```python
from build123d import *

# Parameters (mm, degrees)
SKETCH1_W           = 199.69
SKETCH1_H           = 98.8
SKETCH1_R           = 2
BOSS_EXTRUDE1_DEPTH = 3


with BuildPart() as part:
    # Sketch1 → Boss-Extrude1 (new body)
    with BuildSketch(Plane(origin=(0, 0, 0), x_dir=(1, 0, 0), z_dir=(0, 1, 0))):
        with Locations((49.702752105, -22.572203273)):
            Rectangle(SKETCH1_W, SKETCH1_H)
        with Locations((124.547752105, -0.072203273)):
            Circle(SKETCH1_R, mode=Mode.SUBTRACT)
        with Locations((124.547752105, -45.072203273)):
            Circle(SKETCH1_R, mode=Mode.SUBTRACT)
        with BuildLine():
            Line((-41.155575491, 15.827796727), (3.397752105, 15.827796727))
            ThreePointArc((3.397752105, 15.827796727), (4.281635581, 16.193913251), (4.647752105, 17.077796727))
            Line((4.647752105, 17.077796727), (4.647752105, 17.577796727))
            ThreePointArc((4.647752105, 17.577796727), (5.013868628, 18.461680204), (5.897752105, 18.827796727))
            Line((5.897752105, 18.827796727), (15.397752105, 18.827796727))
            ThreePointArc((15.397752105, 18.827796727), (16.281635581, 18.461680204), (16.647752105, 17.577796727))
            Line((16.647752105, 17.577796727), (16.647752105, 17.077796727))
            ThreePointArc((16.647752105, 17.077796727), (17.013868628, 16.193913251), (17.897752105, 15.827796727))
            Line((17.897752105, 15.827796727), (106.2510797, 15.827796727))
            ThreePointArc((106.2510797, 15.827796727), (107.693618601, 15.253929592), (108.347752105, 13.845969603))
            Line((108.347752105, 13.845969603), (109.547752105, -7.444930545))
            Line((109.547752105, -7.444930545), (109.547752105, -12.572203273))
            ThreePointArc((109.547752105, -12.572203273), (110.71932498, -15.400630397), (113.547752105, -16.572203273))
            Line((113.547752105, -16.572203273), (136.547694997, -16.572203273))
            Line((136.547694997, -16.572203273), (136.547694997, -28.572203273))
            Line((136.547694997, -28.572203273), (113.547752105, -28.572203273))
            ThreePointArc((113.547752105, -28.572203273), (110.71932498, -29.743776148), (109.547752105, -32.572203273))
            Line((109.547752105, -32.572203273), (109.547752105, -37.699476))
            Line((109.547752105, -37.699476), (108.347752105, -58.990376148))
            ThreePointArc((108.347752105, -58.990376148), (107.693618601, -60.398336137), (106.2510797, -60.972203273))
            Line((106.2510797, -60.972203273), (24.097694997, -60.972203273))
            ThreePointArc((24.097694997, -60.972203273), (23.21381152, -61.338319796), (22.847694997, -62.222203273))
            Line((22.847694997, -62.222203273), (22.847694997, -62.722203273))
            ThreePointArc((22.847694997, -62.722203273), (22.481578473, -63.606086749), (21.597694997, -63.972203273))
            Line((21.597694997, -63.972203273), (2.097694997, -63.972203273))
            ThreePointArc((2.097694997, -63.972203273), (1.21381152, -63.606086749), (0.847694997, -62.722203273))
            Line((0.847694997, -62.722203273), (0.847694997, -62.222203273))
            ThreePointArc((0.847694997, -62.222203273), (0.481578473, -61.338319796), (-0.402305003, -60.972203273))
            Line((-0.402305003, -60.972203273), (-41.155575491, -60.972203273))
            ThreePointArc((-41.155575491, -60.972203273), (-42.598114392, -60.398336137), (-43.252247895, -58.990376148))
            Line((-43.252247895, -58.990376148), (-44.452247895, -37.699476))
            Line((-44.452247895, -37.699476), (-44.452247895, -7.444930545))
            Line((-44.452247895, -7.444930545), (-43.252247895, 13.845969603))
            ThreePointArc((-43.252247895, 13.845969603), (-42.598114392, 15.253929592), (-41.155575491, 15.827796727))
        make_face(mode=Mode.SUBTRACT)
    extrude(amount=BOSS_EXTRUDE1_DEPTH)


solid = part.part
```
Build history of the part. All positions in model axes, mm. A direction names the side the tool comes from. Give positions to 0.01 mm unless a question says otherwise; leave off trailing zeros. Loops run counter-clockwise (first coordinate to the right, second up) from the corner with the lowest first, then second, coordinate; pieces in that order, holes last. Notation, with made-up numbers: (66.5, 29) -> (118.5, 29) arc R18 cw to (118.5, 48) -> close; hole circle Ø11 at (13.25, 70.5). An arc over 180 degrees is marked (long way). One line per question, with ' | ' between items. Start each with the question number.
1) Cut at C-C (y = 0.95). Count the separate pieces of the cut face and the enclosed holes in it, plus the area to 3 significant figures.
2) Two-plate mould, pull along X, no slides. Class faces 3 (the flat face through (115, 3, 11)), 4 (the cylindrical face through (126.395, 1.479, 45.838)), 5 (the cylindrical face through (126.455, 1.479, -0.529)): released by +X, released by -X, zero draft, split by the parting line, or undercut.
3) Cut at A-A (z = 25). Give the cut face in (x, y).
4) Cut at B-B (x = 87). Give the cut face in (y, z).
5) Probe L1, parallel to Z at x = -29, y = 2.55; L2, parallel to Z at x = 7, y = 0.7; L3, parallel to X at y = 2.1, z = -1.5. List the from-to ranges inside material, lowest first.
6) Pin check, flat tip, straight feed: pin 1 (2.5 mm diameter, centred on x = 124.55, z = 45.07, fed in from +Y). Stop position of the tip, or through.
7) 3-axis set-ups, long thin cutter, end or side, ignore diameter. For faces 1 (the cylindrical face through (110.751, 1.479, 29.713)), 2 (the flat face through (115, 0, 11)): which of +Z, -Z, +X, -X, +Y, -Y reach the whole face in a straight line?
Return value:
1) separate pieces: 1 | enclosed holes: 3 | area: 7,510 mm^2
2) face 3: zero draft | face 4: undercut | face 5: undercut
3) outline: (-50.14, 0) -> (-44.45, 0) -> (-44.45, 3) -> (-50.14, 3) -> close; (136.55, 0) -> (149.55, 0) -> (149.55, 3) -> (136.55, 3) -> close
4) outline: (0, -26.83) -> (3, -26.83) -> (3, -15.83) -> (0, -15.83) -> close; (0, 60.97) -> (3, 60.97) -> (3, 71.97) -> (0, 71.97) -> close
5) L1: -26.83 to -15.83, 60.97 to 71.97 | L2: -26.83 to -18.83, 63.97 to 71.97 | L3: -50.14 to -43.95, 109.04 to 123.31, 125.78 to 149.55
6) pin 1: through
7) face 1: +Y, -Y | face 2: +Z, -Z, +X, -X, -Y
